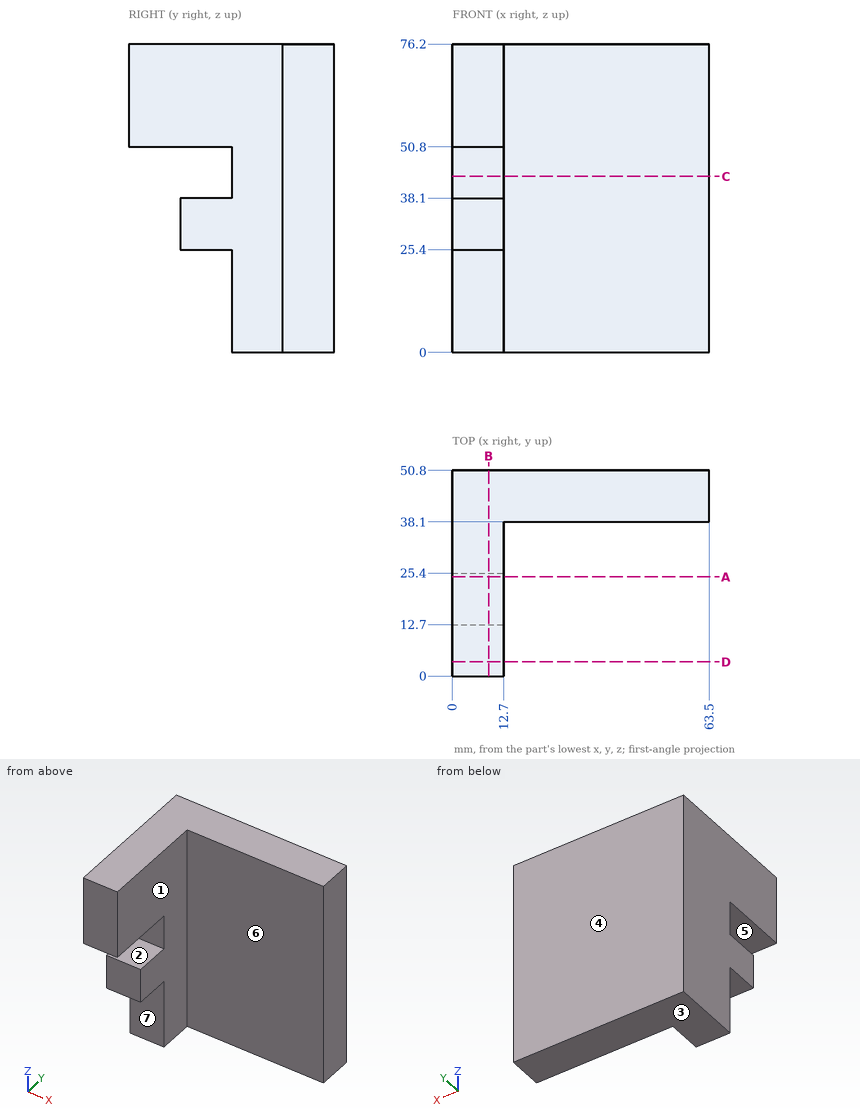
Answer from the drawing. Dimensions are ordinates in mm from the lowest x, y and z of the part. A direction names the side the tool comes from. Coordinates: 2 decimals unless noted, no trailing zeros. Loops run counter-clockwise (first coordinate to the right, second up) from the corner with the lowest first, then second, coordinate; pieces in that order, holes last.
1) Section D-D (y = 3.5) is taken. Give the vertices of the cut face in (x, z).
Results:
outline: (0, 50.8) - (12.7, 50.8) - (12.7, 76.2) - (0, 76.2) - close
2) Consider probe 1 along Z at (x, y) = (10.5, 23.5); probe 2 along X at (y, z) = (30.5, 64); probe 3 along Y at (x, z) = (16.5, 13). Determine where each line is inside the solid, lowest interval first.
Results:
probe 1: z = 25.4 to 38.1, 50.8 to 76.2
probe 2: x = 0 to 12.7
probe 3: y = 38.1 to 50.8
3) For the marked faces 4, 5, 6 and 7, determine the directions among +Z, -Z, +X, -X, +Y, -Y from which every point of the face is accessible in a straight line to the end or side of a thin tool.
Results:
face 4: +Z, -Z, +X, -X, +Y
face 5: +X, -X, -Y
face 6: +Z, -Z, +X, -Y
face 7: -Z, +X, -X, -Y
4) Flat-ended cylindrical pins translate along their axes: pin 1 (4 mm diameter, centred on x = 5.5, z = 44, fed in from -Y); pin 2 (15 mm diameter, centred on x = 26, z = 35.5, fed in from -Y); pin 3 (6.5 mm diameter, centred on x = 3.5, y = 16.5, fed in from -Z). Find the tip coordinate at first contact, or state that the pin passes through.
Results:
pin 1: stops at y = 25.4
pin 2: stops at y = 38.1
pin 3: stops at z = 25.4
5) For a pull along Z with two mould halves and no side action, classify the marked faces 1, 2 and 3 as +Z half, -Z half, draft (parallel to the pull), parting line (faces both ways), or undercut.
Results:
face 1: draft
face 2: undercut
face 3: -Z half
6) Section B-B (x = 9) is taken. Give the vertices of the cut face in (y, z), plus the area to 3 significant figures.
Results:
outline: (0, 50.8) - (25.4, 50.8) - (25.4, 38.1) - (12.7, 38.1) - (12.7, 25.4) - (25.4, 25.4) - (25.4, 0) - (50.8, 0) - (50.8, 76.2) - (0, 76.2) - close
area: 2,740 mm2
7) Section C-C (z = 43.5) is taken. Give the vertices of the cut face in (x, y), plus the area to 3 significant figures.
Results:
outline: (0, 25.4) - (12.7, 25.4) - (12.7, 38.1) - (63.5, 38.1) - (63.5, 50.8) - (0, 50.8) - close
area: 968 mm2
8) Section A-A (y = 24.5) is taken. Give the vertices of the cut face in (x, z), plus the area to 3 significant figures.
Results:
outline: (0, 25.4) - (12.7, 25.4) - (12.7, 38.1) - (0, 38.1) - close; (0, 50.8) - (12.7, 50.8) - (12.7, 76.2) - (0, 76.2) - close
area: 484 mm2
